Input: part model. Units: mm. Frame: model coordinates. Round coordinates to 2 decimals unless told otherwise and drop trailing zeros. Loops run counter-clockwise (first coordinate to the right, second up) from the corner with the lowest first, then second, coordinate; pieces in that order, holes last. Notation, with made-up numbers: M -38.75,16.25 L 13.25,16.25 A21 ccw 13.25,38.25 Z; hole C 88,-25.5 d10. An arc over 180 degrees is marked long. Return JSON: item names as keys, results as strings. Group by question number.
1) Section B-B (z = 5). Output: boundary loops of the cut face in (x, y), plus the area to 3 significant figures.
2) Material intervals for line 1 (Z direction, x = 805.5, y = -21); line 2 (Y direction, x = 625.5, z = -10); line 3 (Y direction, x = 1222, z = 29.85), sorted ascending. Write a range as from..to.
3) Section A-A (x = 935.5). Output: boundary loops of the cut face in (y, z), plus the area to 3 significant figures.
4) Contact query for flat-ended pins moving along their axis: P1, Ø6, axis at x = 1227, y = -23, coming from the -Z side; P2, Ø6, axis at x = 552, y = -5.5, coming from the +Z side; P3, Ø1.5, axis at x = 604, y = -16, coming from the -Z side; P4, Ø12, axis at y = -17, z = 20, coming from the -X side. Output: stop coordinate, or through.
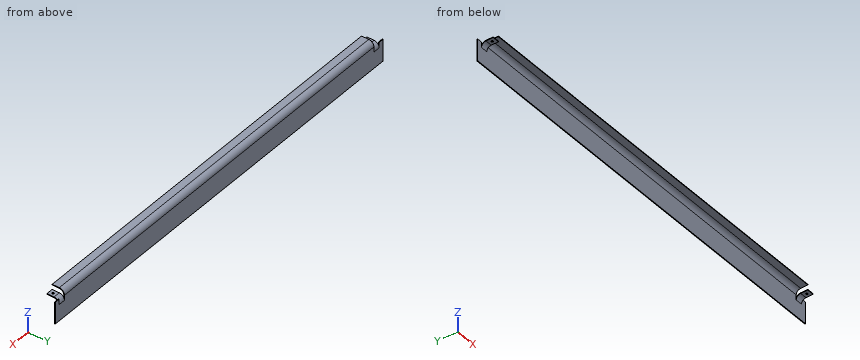
from build123d import *

# Parameters (mm, degrees)
F0_W      = 2
F0_H      = 64
F1_DEPTH  = 15
F3_DEPTH  = 20
F5_DEPTH  = 1177
F7_DEPTH  = 20
F8_W      = 2
F8_H      = 64
F9_DEPTH  = 15
F10_R     = 3
F11_DEPTH = 2
F12_R     = 3
F13_DEPTH = 2


with BuildPart() as f1:
    # F0 (on Right) → F1 (new body)
    with BuildSketch(Plane.YZ):
        Rectangle(F0_W, F0_H)
    extrude(amount=F1_DEPTH)



with BuildPart() as f3:
    # F2 (on face) → F3 (new body)
    with BuildSketch(Plane.YZ.offset(1212)):
        with BuildLine():
            Line((-1, -32), (1, -32))
            Line((1, -32), (1, 16))
            ThreePointArc((1, 16), (-3.393398, 26.606602), (-14, 31))
            Line((-14, 31), (-35, 31))
            Line((-35, 31), (-35, 29))
            Line((-35, 29), (-14, 29))
            ThreePointArc((-14, 29), (-4.807612, 25.192388), (-1, 16))
            Line((-1, 16), (-1, -32))
        make_face()
    extrude(amount=F3_DEPTH)

    # F4 (on face) → F5 (join)
    with BuildSketch(Plane.YZ.offset(35)):
        with BuildLine():
            Line((-1, -32), (1, -32))
            Line((1, -32), (1, 31))
            ThreePointArc((1, 31), (-3.393398, 41.606602), (-14, 46))
            Line((-14, 46), (-35, 46))
            Line((-35, 46), (-35, 44))
            Line((-35, 44), (-14, 44))
            ThreePointArc((-14, 44), (-4.807612, 40.192388), (-1, 31))
            Line((-1, 31), (-1, -32))
        make_face()
    extrude(amount=F5_DEPTH)


with BuildPart() as f1_1:
    add(f1.part)

    add(f3.part)  # F7 merges F3
    # F6 (on face) → F7 (join)
    with BuildSketch(Plane.YZ.offset(15)):
        with BuildLine():
            Line((-1, -32), (1, -32))
            Line((1, -32), (1, 16))
            ThreePointArc((1, 16), (-3.393398, 26.606602), (-14, 31))
            Line((-14, 31), (-35, 31))
            Line((-35, 31), (-35, 29))
            Line((-35, 29), (-14, 29))
            ThreePointArc((-14, 29), (-4.807612, 25.192388), (-1, 16))
            Line((-1, 16), (-1, -32))
        make_face()
    extrude(amount=F7_DEPTH)

    # F8 (on face) → F9 (join)
    with BuildSketch(Plane.YZ.offset(1232)):
        Rectangle(F8_W, F8_H)
    extrude(amount=F9_DEPTH)

    # F10 (on face) → F11 (cut)
    with BuildSketch(Plane.XY.offset(31)):
        with Locations((1222, -24.5)):
            Circle(F10_R)
    extrude(amount=-F11_DEPTH, mode=Mode.SUBTRACT)

    # F12 (on face) → F13 (cut)
    with BuildSketch(Plane.XY.offset(31)):
        with Locations((25, -24.5)):
            Circle(F12_R)
    extrude(amount=-F13_DEPTH, mode=Mode.SUBTRACT)


solid = f1_1.part
Returned:
{
 "1": {"outline": "M 0,-1 L 1247,-1 L 1247,1 L 0,1 Z", "area": "2,490 mm^2"},
 "2": {"line 1": "z = 44..46", "line 2": "y = -1..1", "line 3": "y = -35..-27.5, -21.5..-8.24"},
 "3": {"outline": "M -35,44 L -14,44 A13 cw -1,31 L -1,-32 L 1,-32 L 1,31 A15 ccw -14,46 L -35,46 Z", "area": "212 mm^2"},
 "4": {"P1": "stops at z = 29", "P2": "stops at z = 44.96", "P3": "stops at z = 44", "P4": "passes through"}
}
